```python
from build123d import *

# Parameters (mm, degrees)
SKETCH_1_R               = 4.5
EXTRUDE_2_DEPTH          = 33
CUT_EXTRUDE_3_DEPTH      = 42
SKETCH_6_W               = 24
SKETCH_6_H               = 12
CUT_EXTRUDE_4_DEPTH      = 85.587779831
CUT_EXTRUDE_5_DEPTH      = 85.587779831
CUT_EXTRUDE_5_DEPTH_BACK = 85.587779831
SKETCH_7_W               = 78
SKETCH_7_H               = 9
CUT_EXTRUDE_6_DEPTH      = 85.587779831
CUT_EXTRUDE_6_DEPTH_BACK = 85.587779831
SKETCH_8_W               = 42
SKETCH_8_H               = 6
SKETCH_8_H_2             = 3
CUT_EXTRUDE_7_DEPTH      = 105.787400596
CUT_EXTRUDE_7_DEPTH_BACK = 105.787400596
SKETCH_9_R               = 3


with BuildPart() as part:
    # 草图1 → 凸台-拉伸2 (new body)
    with BuildSketch(Plane.XY):
        with BuildLine():
            Line((52.828829832, 42.32492556), (52.828829832, 27.32492556))
            ThreePointArc((52.828829832, 27.32492556), (51.828829832, 9.38065365), (50.828829832, 27.32492556))
            Line((50.828829832, 27.32492556), (50.828829832, 42.32492556))
            Line((50.828829832, 42.32492556), (36.828829832, 42.32492556))
            Line((36.828829832, 42.32492556), (36.828829832, 2.32492556))
            Line((36.828829832, 2.32492556), (-11.171170168, 2.32492556))
            Line((-11.171170168, 2.32492556), (-11.171170168, -15.67507444))
            Line((-11.171170168, -15.67507444), (-35.171170168, -15.67507444))
            Line((-35.171170168, -15.67507444), (-35.171170168, 12.32492556))
            ThreePointArc((-35.171170168, 12.32492556), (-44.171170168, 21.32492556), (-53.171170168, 12.32492556))
            Line((-53.171170168, 12.32492556), (-53.171170168, -15.67507444))
            ThreePointArc((-53.171170168, -15.67507444), (-47.899092229, -28.402996501), (-35.171170168, -33.67507444))
            Line((-35.171170168, -33.67507444), (34.828829832, -33.67507444))
            ThreePointArc((34.828829832, -33.67507444), (57.45624683, -24.302491437), (66.828829832, -1.67507444))
            Line((66.828829832, -1.67507444), (66.828829832, 42.32492556))
            Line((66.828829832, 42.32492556), (52.828829832, 42.32492556))
        make_face()
        with Locations((-44.171170168, 12.32492556)):
            Circle(SKETCH_1_R, mode=Mode.SUBTRACT)
    extrude(amount=EXTRUDE_2_DEPTH)

    # 草图4 → 切除-拉伸3 (cut)
    with BuildSketch(Plane.ZY.offset(53.171170168)):
        Polygon((0, 0.32492556), (18, -15.67507444), (18, -33.67507444), (0, -33.67507444), align=None)
        Polygon((15, 21.32492556), (15, 3.32492556), (33, -12.67507444), (33, 21.32492556), align=None)
    extrude(amount=-CUT_EXTRUDE_3_DEPTH, mode=Mode.SUBTRACT)

    # 草图6 → 切除-拉伸4 (cut, through all)
    with BuildSketch(Plane(origin=(0, 2.32492556, 0), x_dir=(1, 0, 0), z_dir=(0, 1, 0))):
        with Locations((6.828829832, -21)):
            Rectangle(SKETCH_6_W, SKETCH_6_H)
    extrude(amount=-CUT_EXTRUDE_4_DEPTH, mode=Mode.SUBTRACT)

    # 草图7 → 切除-拉伸5 (cut, two sides: drawn at the far end of the back side and taken through both)
    with BuildSketch(Plane(origin=(0, 2.32492556, 0), x_dir=(1, 0, 0), z_dir=(0, 1, 0)).offset(-CUT_EXTRUDE_5_DEPTH_BACK)):
        with Locations((27.828829832, -4.5)):
            Rectangle(SKETCH_7_W, SKETCH_7_H)
    extrude(amount=CUT_EXTRUDE_5_DEPTH + CUT_EXTRUDE_5_DEPTH_BACK, mode=Mode.SUBTRACT)

    # 草图8 → 切除-拉伸6 (cut, two sides: drawn at the far end of the back side and taken through both)
    with BuildSketch(Plane(origin=(0, 2.32492556, 0), x_dir=(1, 0, 0), z_dir=(0, 1, 0)).offset(-CUT_EXTRUDE_6_DEPTH_BACK)):
        with Locations((45.828829832, -12)):
            Rectangle(SKETCH_8_W, SKETCH_8_H)
        with Locations((45.828829832, -31.5)):
            Rectangle(SKETCH_8_W, SKETCH_8_H_2)
    extrude(amount=CUT_EXTRUDE_6_DEPTH + CUT_EXTRUDE_6_DEPTH_BACK, mode=Mode.SUBTRACT)

    # 草图9 → 切除-拉伸7 (cut, two sides: drawn at the far end of the back side and taken through both)
    with BuildSketch(Plane.ZY.offset(-36.828829832).offset(-CUT_EXTRUDE_7_DEPTH_BACK)):
        with Locations(Location((22.5, 36.32492556, 0), (0, 0, 270))):
            Circle(SKETCH_9_R)
    extrude(amount=CUT_EXTRUDE_7_DEPTH + CUT_EXTRUDE_7_DEPTH_BACK, mode=Mode.SUBTRACT)


solid = part.part
```
Verification items for the finished model (mm, model axes). A direction names the side the tool comes from. Round coordinates to 2 decimals unless told otherwise and drop trailing zeros. Write each loop counter-clockwise with the first axis right and the second up, starting at its lowest first coordinate (ties: lowest second). Pieces come first, ordered by that corner, then holes. Notation, with made-up numbers: (15, 41) -> (62, 41) arc R22 ccw to (62, 78) -> close; hole circle Ø2 at (70.25, 18). An arc over 180 degrees is marked (long way). Write each question's results on one line, items separated by ' | '.
Q1. Go/stop test with flat-tipped pins: pin 1 Ø2 at (x, y) = (42, 32.5) entering from +Z; pin 2 Ø14.5 at (x, y) = (-44.17, 12.32) entering from +Z; pin 3 Ø6 at (y, z) = (-22.5, 19) entering from -X; pin 4 Ø14.5 at (x, y) = (51.83, 18.38) entering from +Z. Record where each tip stops, or that it passes through.
Derived:
pin 1: stops at z = 30 | pin 2: stops at z = 15 | pin 3: stops at x = -52.76 | pin 4: passes through
Q2. Sectioned sample at C-C, the plane y = -8. Record the boundary of the cut face in (x, z), and give its area (3 significant figures).
Derived:
outline: (-53.17, 9.37) -> (-35.17, 9.37) -> (-35.17, 27.74) -> (-53.17, 27.74) -> close; (-11.17, 9) -> (24.83, 9) -> (24.83, 15) -> (66.2, 15) -> (66.2, 30) -> (24.83, 30) -> (24.83, 33) -> (-11.17, 33) -> close; hole (-5.17, 15) -> (18.83, 15) -> (18.83, 27) -> (-5.17, 27) -> close | area: 1,530 mm²
Q3. Sectioned sample at A-A, the plane x = -3.5. Record the boundary of the cut face in (y, z), and give its area (3 significant figures).
Derived:
outline: (-33.68, 9) -> (2.32, 9) -> (2.32, 15) -> (-33.68, 15) -> close; (-33.68, 27) -> (2.32, 27) -> (2.32, 33) -> (-33.68, 33) -> close | area: 432 mm²
Q4. Sectioned sample at B-B, the plane z = 13.5. Record the boundary of the cut face in (x, y).
Derived:
outline: (-53.17, -11.68) -> (-35.17, -11.68) -> (-35.17, 12.32) arc R9 ccw to (-53.17, 12.32) -> close; (-11.17, -33.68) -> (24.83, -33.68) -> (24.83, 2.32) -> (-11.17, 2.32) -> close; hole circle Ø9 at (-44.17, 12.32)
Q5. Thickness scan on probe 1 along X at (y, z) = (1.5, 17); probe 2 along X at (y, z) = (28.5, 29); probe 3 along Z at (x, y) = (3.5, -23.5). Record the ranges inside material, lowest first.
Derived:
probe 1: x = -53.17 to -35.17, -11.17 to -5.17, 18.83 to 66.83 | probe 2: x = 36.83 to 50.83, 52.83 to 66.83 | probe 3: z = 9 to 15, 27 to 33
Q6. Draft check along Y on faces 5 (the face through (-35.171, -2, 16)), 6 (the face through (59.927, 33.463, 23.401)), 7 (the face through (60, 42.325, 22)). Enter one of: released by +Y, released by -Y, zero draft, split by the parting line, or undercut.
Derived:
face 5: zero draft | face 6: undercut | face 7: released by +Y
Q7. Sectioned sample at D-D, the plane z = 22.5. Record the boundary of the cut face in (x, y), and give its area (3 significant figures).
Derived:
outline: (-53.17, -15.68) arc R18 ccw to (-35.17, -33.68) -> (-5.17, -33.68) -> (-5.17, 2.32) -> (-11.17, 2.32) -> (-11.17, -15.68) -> (-35.17, -15.68) -> (-35.17, -3.34) -> (-53.17, -3.34) -> close; (18.83, -33.68) -> (34.83, -33.68) arc R32 ccw to (66.83, -1.68) -> (66.83, 33.32) -> (52.83, 33.32) -> (52.83, 27.32) arc R9 cw (long way) to (50.83, 27.32) -> (50.83, 33.32) -> (36.83, 33.32) -> (36.83, 2.32) -> (18.83, 2.32) -> close; (36.83, 39.32) -> (50.83, 39.32) -> (50.83, 42.32) -> (36.83, 42.32) -> close; (52.83, 39.32) -> (66.83, 39.32) -> (66.83, 42.32) -> (52.83, 42.32) -> close | area: 3,380 mm²
Q8. Access from +Z, -Z, +X, -X, +Y, -Y to the whole of each face (thin tool, end or side, straight path). Record for faces 1 (the face through (24.829, -16, 32)), 2 (the face through (-32, -25, 18)), 3 (the face through (13, 2.325, 29)), 4 (the face through (7, -16, 9)).
Derived:
face 1: +Z, +X, +Y, -Y | face 2: -Z, -X, -Y | face 3: +Z, -Z, +Y | face 4: -Z, +X, +Y, -Y
